Job drawing, mm, ordinate dimensions from the low corner. One solid piece. Give positions to 0.01 mm unless a question says otherwise; leave off trailing zeros. Loops run counter-clockwise (first coordinate to the right, second up) from the corner with the lowest first, then second, coordinate; pieces in that order, holes last. Notation, with made-up numbers: M 59.25,83.5 L 90.25,83.5 A13 ccw 90.25,97.5 Z; hole C 25,-5.75 d8. An arc over 180 degrees is marked long. Put each result on its own line as item: value.
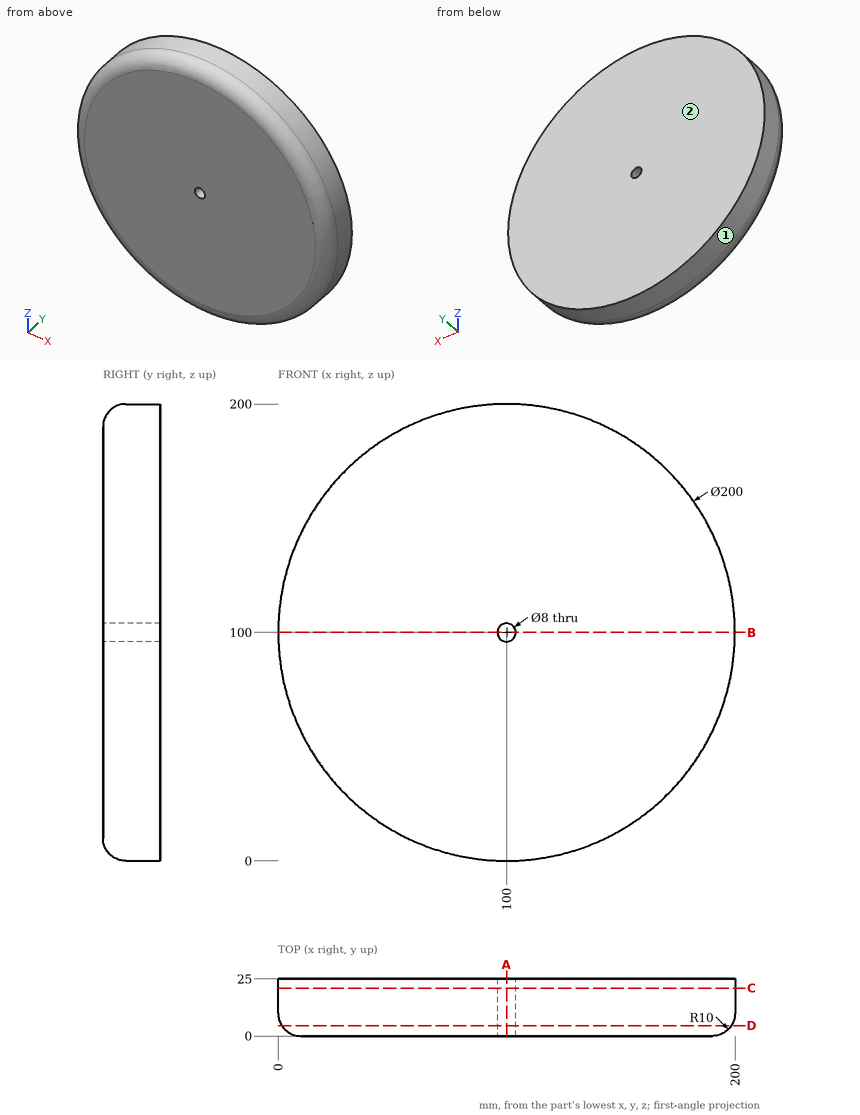
Q1. Mould opens along Z. For the marked faces 1 and 2 say: pulls with the +Z half, pulls with the -Z half, needs draft (parallel to the pull), parting line crosses it, or undercut.
Here are the results:
face 1: parting line crosses it
face 2: needs draft
Q2. Slice it at C-C (y = 21). List the corners of the cut face in (x, z), and give its area (3 significant figures).
Here are the results:
outline: C 100,100 d200; hole C 100,100 d8
area: 31,400 mm²
Q3. Slice it at D-D (y = 4.5). List the corners of the cut face in (x, z).
Here are the results:
outline: C 100,100 d196.7; hole C 100,100 d8
Q4. Slice it at A-A (x = 100). List the corners of the cut face in (y, z).
Here are the results:
outline: M 0,10 A10 ccw 10,0 L 25,0 L 25,96 L 0,96 Z; M 0,104 L 25,104 L 25,200 L 10,200 A10 ccw 0,190 Z
Q5. Drop flat-ended pins along their axis: pin 1 Ø4 at (y, z) = (6, 91) entering from +X; pin 2 Ø5 at (y, z) = (16.5, 52) entering from -X; pin 3 Ø3 at (y, z) = (7.5, 22.5) entering from +X. Give the stop position or say it passes through.
Here are the results:
pin 1: x = 199.43
pin 2: x = 10.95
pin 3: x = 164.58
Q6. Slice it at B-B (z = 100). List the corners of the cut face in (x, y), and give its area (3 significant figures).
Here are the results:
outline: M 0,10 A10 ccw 10,0 L 96,0 L 96,25 L 0,25 Z; M 104,0 L 190,0 A10 ccw 200,10 L 200,25 L 104,25 Z
area: 4,760 mm²
Q7. Probe line 1 (Z direction, x = 100, y = 16); line 2 (Z direction, x = 100, y = 6.25); line 3 (Y direction, x = 181, z = 60). List the from-to ranges inside material, lowest first. Write a range as from..to.
Here are the results:
line 1: 0..96, 104..200
line 2: 0.73..96, 104..199.27
line 3: 0.01..25
